Build history of the part. All positions in model axes, mm. A direction names the side the tool comes from. Round coordinates to 2 decimals unless told otherwise and drop trailing zeros. Loops run counter-clockwise (first coordinate to the right, second up) from the corner with the lowest first, then second, coordinate; pieces in that order, holes last. Notation, with made-up numbers: M 22,53 L 42,53 A28 cw 42,74 Z; hole C -30.75,65 d2. An arc over 180 degrees is marked long. Use one line per item in the form item = value. Start each with the question number.
```python
from build123d import *

# Parameters (mm, degrees)
F1_DEPTH = 22.352
F2_DEPTH = 3.175
F4_DEPTH = 25.4
F5_R     = 6.35
F5_R_2   = 3.175
F6_DEPTH = 3.175
F7_DEPTH = 25.4
F8_R     = 10.922


with BuildPart() as f1:
    # F0 (on Front) → F1 (new body, symmetric)
    with BuildSketch(Plane.XZ):
        Polygon((-34.0286190226, 0), (57.3959515745, 0), (57.3959515745, 9.652), (-3.0560484255, 9.652), (-28.4560484255, 9.652), (-47.5060484255, 42.6475678842), (-55.8726190226, 37.8349178405), align=None)
    extrude(amount=F1_DEPTH, both=True)

    # F0 (on Front) → F2 (join, symmetric)
    with BuildSketch(Plane.XZ):
        Polygon((-28.4560484255, 9.652), (-3.0560484255, 9.652), (-47.5060484255, 42.6475678842), align=None)
    extrude(amount=F2_DEPTH, both=True)

    # F3 (on face) → F4 (cut)
    with BuildSketch(Plane.XY.offset(9.652)):
        with BuildLine():
            ThreePointArc((35.0439515745, 22.352), (57.3043185829, -1.03671e-05), (35.043930755, -22.352))
            Line((35.043930755, -22.352), (57.3959515745, -22.352))
            Line((57.3959515745, -22.352), (57.3959515745, 22.352))
            Line((57.3959515745, 22.352), (35.0439515745, 22.352))
        make_face()
        with BuildLine():
            Line((35.0439515745, 11.176), (9.6439515745, 11.176))
            ThreePointArc((9.6439515745, 11.176), (-1.5320366113, -0.0162502311), (9.6764520023, -11.1759527434))
            Line((9.6764520023, -11.1759527434), (35.043930755, -11.176))
            ThreePointArc((35.043930755, -11.176), (46.2199515745, -1.04098e-05), (35.0439515745, 11.176))
        make_face()
    extrude(amount=-F4_DEPTH, mode=Mode.SUBTRACT)

    # F5 (on face) → F6 (cut)
    with BuildSketch(Plane(origin=(-17.1625977204, 0, -9.9088304139), x_dir=(0, 1, 0), z_dir=(0.8660254038, 0, 0.5))):
        with Locations((11.43, 49.7649014101)):
            Circle(F5_R)
        with Locations((11.43, 49.7649014101)):
            Circle(F5_R_2, mode=Mode.SUBTRACT)
        with Locations((-11.43, 49.7649014101)):
            Circle(F5_R)
        with Locations((-11.43, 49.7649014101)):
            Circle(F5_R_2, mode=Mode.SUBTRACT)
    extrude(amount=-F6_DEPTH, mode=Mode.SUBTRACT)

    # F7 (cut): faces of the model
    f7_faces = [f1.faces().sort_by_distance(p)[0] for p in [
        (-42.0450484255, -11.43, 33.1888384241),
        (-42.0450484255, 11.43, 33.1888384241),
    ]]
    extrude(f7_faces, amount=-F7_DEPTH, mode=Mode.SUBTRACT)

    # F8
    f8_edges = [f1.edges().sort_by_distance(p)[0] for p in [
        (-51.689334, -22.352, 40.241243),
        (-51.689334, 22.352, 40.241243),
    ]]
    fillet(f8_edges, radius=F8_R)


solid = f1.part
```
Q1. Saw through at D-D (x = -5). Give the cut face in (y, z) (3 decimals).
Q2. Saw through at A-A (y = 0). Give the cut face in (x, z).
Q3. Wall check: probe 1 along Y at (x, z) = (-43, 29); probe 2 along Y at (x, z) = (25, 4.5); probe 3 along Z at (x, y) = (-21.5, -11.5). Give the ranges that are in metal, low to high.
Q4. Pull direction Y, two halves, no side cores. Call faces 5 (the face through (-25, 3.175, 20)), 6 (the face through (-50.103, -19.237, 37.365)), 7 (the face through (-40.3, 10.05, 27.04)): pulls with the +Y half, pulls with the -Y half, needs draft (parallel to the pull), parting line crosses it, or undercut.
Q5. Tool access for faces 1 (the face through (-35.73, 12.63, 22.25)), 2 (the face through (-25, -3.175, 20)), 3 (the face through (-43.428, 14.163, 29.234)), 4 (the face through (46.217, -0.246, 4.894)): list every direction of +Z, -Z, +X, -X, +Y, -Y with a clear straight run to the whole face (end or side of a thin tool).
Q6. Saw through at C-C (z = 8.5). Give the cut face in (x, y), and give its area (3 significant figures).
Q7. Saw through at B-B (z = 16). Give the cut face in (x, y) (3 decimals), and give its area (3 significant figures).
Q8. Drop flat-ended pins along their axis: P1, Ø4, axis at x = -6, y = -3, coming from the +Z side; P2, Ø10, axis at x = 26, y = 4.5, coming from the -Z side; P3, Ø12, axis at y = 14.5, z = 32, coming from the -X side; P4, Ø4, axis at x = -31.5, z = 29.5, coming from the +Y side (3 decimals). Give the stop position or say it passes through.
Filled in:
q1.outline = M -22.352,0 L 22.352,0 L 22.352,9.652 L 3.175,9.652 L 3.175,11.095 L -3.175,11.095 L -3.175,9.652 L -22.352,9.652 Z
q2.outline = M -55.87,37.83 L -34.03,0 L -1.53,0 L -1.53,9.65 L -3.06,9.65 L -47.51,42.65 Z; M 46.22,0 L 57.3,0 L 57.3,9.65 L 46.22,9.65 Z
q3.probe_1 = -22.35 to -16.94, -5.92 to 5.92, 16.94 to 22.35
q3.probe_2 = -22.35 to -11.18, 11.18 to 22.35
q3.probe_3 = 0 to 9.65
q4.face_5 = pulls with the +Y half
q4.face_6 = pulls with the -Y half
q4.face_7 = undercut
q5.face_1 = +Z, +X, +Y
q5.face_2 = +Z, +X, -Y
q5.face_3 = none
q5.face_4 = +Z, -Z
q6.outline = M -38.94,-22.35 L 35.04,-22.35 A22.35 ccw 35.04,22.35 L -38.94,22.35 Z; hole M 9.64,11.18 A11.18 ccw 9.68,-11.18 L 35.04,-11.18 A11.18 ccw 35.04,11.18 Z
q6.area = 3,130 mm²
q7.outline = M -43.266,-22.352 L -32.121,-22.352 L -32.121,-3.175 L -11.608,-3.175 L -11.608,3.175 L -32.121,3.175 L -32.121,22.352 L -43.266,22.352 Z
q7.area = 628 mm²
q8.P1 = 13.32
q8.P2 = through
q8.P3 = -55.83
q8.P4 = 3.175
